from build123d import *

# Parameters (mm, degrees)
F0_W          = 73.54109
F0_H          = 45.764141
F1_DEPTH      = 12.7
F1_DEPTH_BACK = 12.7
F2_R          = 8.170482
F3_DEPTH      = 25.4
F4_R          = 9.904199
F5_DEPTH      = 25.4
F6_R          = 7.936434
F7_DEPTH      = 25.4
F8_R          = 7.144879
F9_DEPTH      = 25.4


with BuildPart() as f1:
    # F0 (on Top) → F1 (new body, two sides)
    with BuildSketch(Plane.XY) as f1_sk:
        with Locations((0.04258, 2.530917)):
            Rectangle(F0_W, F0_H)
    extrude(amount=F1_DEPTH)
    extrude(f1_sk.sketch, amount=-F1_DEPTH_BACK)

    # F2 (on face) → F3 (join)
    with BuildSketch(Plane(origin=(0, 0, -12.7), x_dir=(1, 0, 0), z_dir=(0, 0, -1))):
        with Locations((23.680719, 10.929562)):
            Circle(F2_R)
    extrude(amount=F3_DEPTH)

    # F4 (on face) → F5 (join)
    with BuildSketch(Plane(origin=(0, 0, -12.7), x_dir=(1, 0, 0), z_dir=(0, 0, -1))):
        with Locations((19.757286, -11.209806)):
            Circle(F4_R)
    extrude(amount=F5_DEPTH)

    # F6 (on face) → F7 (join)
    with BuildSketch(Plane(origin=(0, 0, -12.7), x_dir=(1, 0, 0), z_dir=(0, 0, -1))):
        with Locations((-20.317776, 9.248092)):
            Circle(F6_R)
    extrude(amount=F7_DEPTH)

    # F8 (on face) → F9 (join)
    with BuildSketch(Plane(origin=(0, 0, -12.7), x_dir=(1, 0, 0), z_dir=(0, 0, -1))):
        with Locations((-13.031401, -6.44564)):
            Circle(F8_R)
    extrude(amount=F9_DEPTH)


solid = f1.part
Work out the finished part from the listing and answer in its coordinate system (mm). A direction names the side the tool comes from. Give positions to 0.01 mm unless a question says otherwise; leave off trailing zeros. Order: outer loops, then holes, each group sorted by start corner. A loop starts at its lowest first (then second) coordinate and runs counter-clockwise, first axis right, second up. Notation, with made-up numbers: (79, 76) -> (120, 76) arc R17 ccw to (120, 91) -> close; hole circle Ø9 at (24.5, 30). An arc over 180 degrees is marked (long way). Answer as a JSON object with one key per item and string values. Group by question number.
1. Section C-C on z = -34 is taken. Determine the outline of the cut face in (x, y).
2. Flat-ended cylindrical pins translate along their axes: pin 1 Ø5 at (x, y) = (-1, 5) entering from -Z; pin 2 Ø1 at (y, z) = (3.5, -29.5) entering from -X; pin 3 Ø5 at (y, z) = (19.5, -26) entering from -X. Find the tip coordinate at first contact, or state that the pin passes through.
3. Consider line 1 along Z through (x, y) = (15.5, 0.5); line 2 along Y through (x, z) = (-19, -17.5); line 3 along X through (y, z) = (-8, -13). Determine where each line is inside the solid, lowest interval first. Write a range as [from, to].
4. The mould has two halves that part along Y. Classify faces 3 (the cylindrical face through (31.23, -7.8, -25.22)), 4 (the cylindrical face through (-9.73, 12.78, -25.22)), 5 (the flat face through (0, -20.351, 0)), 6 (the flat face through (0, 3, 12.7)): released by +Y, released by -Y, zero draft, split by the parting line, or undercut.
5. Section A-A on x = -15.5 is taken. Determine the outline of the cut face in (y, z), plus the area to 3 significant figures.
6. Section B-B on y = 19.5 is taken. Determine the outline of the cut face in (x, z), plus the area to 3 significant figures.
7. Section D-D on x = 18 is taken. Determine the outline of the cut face in (y, z).
8. A tool of negligible diameter and unlimited length cuts with its end or side. For faces 1 (the flat face through (0, 25.413, 0)), 2 (the flat face through (0, 3, -12.7)), from which of +Z, -Z, +X, -X, +Y, -Y can it reach the whole face along a straight path? Write none if from no direction.
Result sheet:
{
 "1": {"outline": "circle Ø15.87 at (-20.32, -9.25); circle Ø14.29 at (-13.03, 6.45); circle Ø19.81 at (19.76, 11.21); circle Ø16.34 at (23.68, -10.93)"},
 "2": {"pin 1": "stops at z = -12.7", "pin 2": "stops at x = -19.74", "pin 3": "stops at x = 11.72"},
 "3": {"line 1": "z = [-12.7, 12.7]", "line 2": "y = [-17.07, -1.42], [2.52, 10.37]", "line 3": "x = [-28.16, -12.48], [16.05, 31.31]"},
 "4": {"face 3": "undercut", "face 4": "undercut", "face 5": "released by -Y", "face 6": "zero draft"},
 "5": {"outline": "(-20.35, -12.7) -> (-15.55, -12.7) -> (-15.55, -38.1) -> (-2.94, -38.1) -> (-2.94, -12.7) -> (-0.26, -12.7) -> (-0.26, -38.1) -> (13.15, -38.1) -> (13.15, -12.7) -> (25.41, -12.7) -> (25.41, 12.7) -> (-20.35, 12.7) -> close", "area": "1,820 mm^2"},
 "6": {"outline": "(-36.73, -12.7) -> (14.34, -12.7) -> (14.34, -38.1) -> (25.18, -38.1) -> (25.18, -12.7) -> (36.81, -12.7) -> (36.81, 12.7) -> (-36.73, 12.7) -> close", "area": "2,140 mm^2"},
 "7": {"outline": "(-20.35, -12.7) -> (-16.8, -12.7) -> (-16.8, -38.1) -> (-5.06, -38.1) -> (-5.06, -12.7) -> (1.46, -12.7) -> (1.46, -38.1) -> (20.96, -38.1) -> (20.96, -12.7) -> (25.41, -12.7) -> (25.41, 12.7) -> (-20.35, 12.7) -> close"},
 "8": {"face 1": "+Z, -Z, +X, -X, +Y", "face 2": "-Z"}
}
